Build history of the part. All positions in model axes, mm. A direction names the side the tool comes from. Give positions to 0.01 mm unless a question says otherwise; leave off trailing zeros. Loops run counter-clockwise (first coordinate to the right, second up) from the corner with the lowest first, then second, coordinate; pieces in that order, holes last.
1) Band-saw the part on C-C on y = 1. List the corners of the cut face in (x, z), then the cut area to 3 significant figures.
2) Flat gauge pin, fed straight in: P1, Ø5.5, axis at x = -3.5, y = -0.5, coming from the +Z side. Where does the tip first touch, or does it go through?
3) Band-saw the part on B-B on x = 4.5. List the corners of the cut face in (y, z).
4) Band-saw the part on D-D on z = 6.75. List the corners of the cut face in (x, y).
5) 3-axis set-ups, long thin cutter, end or side, ignore diameter. For faces 4 (the cylindrical face through (9.644, 6.124, 4.19)), 5 (the flat face through (-8.5, 0, 4)): which of +Z, -Z, +X, -X, +Y, -Y reach the whole face in a straight line?
6) Two-plate mould, pull along Y, no slides. Class faces 1 (the cylindrical face through (-9.644, -6.124, 4.19)), 2 (the flat face through (0, -5, 4)), 3 (the flat face through (0, 6.5, 4)): +Y half, -Y half, draft (parallel to the pull), parting line (faces both ways), or undercut.
7) Band-saw the part on A-A on z = 4.25. List the corners of the cut face in (x, y), then the cut area to 3 significant figures.
8) Wall check: line 1 (Y direction, x = -6, z = 8.25); line 2 (X direction, y = -2, z = 7.75); line 3 (X direction, y = 4.75, z = 3.75). Give the ranges that are in metal, low to high.
```python
from build123d import *

# Parameters (mm, degrees)
F1_DEPTH = 1.5
F3_DEPTH = 7
F5_DEPTH = 2


with BuildPart() as f1:
    # F0 (on Top) → F1 (new body)
    with BuildSketch(Plane.XY):
        with BuildLine():
            Line((8.75, 6.5), (-8.75, 6.5))
            ThreePointArc((-8.75, 6.5), (-9.633883, 6.133883), (-10, 5.25))
            Line((-10, 5.25), (-10, -5.25))
            ThreePointArc((-10, -5.25), (-9.633883, -6.133883), (-8.75, -6.5))
            Line((-8.75, -6.5), (8.75, -6.5))
            ThreePointArc((8.75, -6.5), (9.633883, -6.133883), (10, -5.25))
            Line((10, -5.25), (10, 5.25))
            ThreePointArc((10, 5.25), (9.633883, 6.133883), (8.75, 6.5))
        make_face()
    extrude(amount=F1_DEPTH)

    # F2 (on face) → F3 (join)
    with BuildSketch(Plane.XY.offset(1.5)):
        with BuildLine():
            ThreePointArc((10, 5.25), (9.633883, 6.133883), (8.75, 6.5))
            Line((8.75, 6.5), (-8.75, 6.5))
            ThreePointArc((-8.75, 6.5), (-9.633883, 6.133883), (-10, 5.25))
            Line((-10, 5.25), (-10, -5.25))
            ThreePointArc((-10, -5.25), (-9.633883, -6.133883), (-8.75, -6.5))
            Line((-8.75, -6.5), (8.75, -6.5))
            ThreePointArc((8.75, -6.5), (9.633883, -6.133883), (10, -5.25))
            Line((10, -5.25), (10, 5.25))
        make_face()
        with BuildLine():
            ThreePointArc((-8.5, 3.75), (-8.133883, 4.633883), (-7.25, 5))
            Line((-7.25, 5), (7.25, 5))
            ThreePointArc((7.25, 5), (8.133883, 4.633883), (8.5, 3.75))
            Line((8.5, 3.75), (8.5, -3.75))
            ThreePointArc((8.5, -3.75), (8.133883, -4.633883), (7.25, -5))
            Line((7.25, -5), (-7.25, -5))
            ThreePointArc((-7.25, -5), (-8.133883, -4.633883), (-8.5, -3.75))
            Line((-8.5, -3.75), (-8.5, 3.75))
        make_face(mode=Mode.SUBTRACT)
    extrude(amount=F3_DEPTH)

    # F4 (on face) → F5 (cut)
    with BuildSketch(Plane.XY.offset(8.5)):
        with BuildLine():
            Line((8, 5.5), (-8, 5.5))
            ThreePointArc((-8, 5.5), (-8.707107, 5.207107), (-9, 4.5))
            Line((-9, 4.5), (-9, -4.5))
            ThreePointArc((-9, -4.5), (-8.707107, -5.207107), (-8, -5.5))
            Line((-8, -5.5), (8, -5.5))
            ThreePointArc((8, -5.5), (8.707107, -5.207107), (9, -4.5))
            Line((9, -4.5), (9, 4.5))
            ThreePointArc((9, 4.5), (8.707107, 5.207107), (8, 5.5))
        make_face()
    extrude(amount=-F5_DEPTH, mode=Mode.SUBTRACT)


solid = f1.part
```
Findings below:
1. outline: (-10, 0) - (10, 0) - (10, 8.5) - (9, 8.5) - (9, 6.5) - (8.5, 6.5) - (8.5, 1.5) - (-8.5, 1.5) - (-8.5, 6.5) - (-9, 6.5) - (-9, 8.5) - (-10, 8.5) - close
1. area: 49.0 mm2
2. P1: stops at z = 1.5
3. outline: (-6.5, 0) - (6.5, 0) - (6.5, 8.5) - (5.5, 8.5) - (5.5, 6.5) - (5, 6.5) - (5, 1.5) - (-5, 1.5) - (-5, 6.5) - (-5.5, 6.5) - (-5.5, 8.5) - (-6.5, 8.5) - close
4. outline: (-10, -5.25) arc R1.25 ccw to (-8.75, -6.5) - (8.75, -6.5) arc R1.25 ccw to (10, -5.25) - (10, 5.25) arc R1.25 ccw to (8.75, 6.5) - (-8.75, 6.5) arc R1.25 ccw to (-10, 5.25) - close; hole (-9, -4.5) arc R1 ccw to (-8, -5.5) - (8, -5.5) arc R1 ccw to (9, -4.5) - (9, 4.5) arc R1 ccw to (8, 5.5) - (-8, 5.5) arc R1 ccw to (-9, 4.5) - close
5. face 4: +Z, -Z, +X, +Y
5. face 5: +Z
6. face 1: -Y half
6. face 2: undercut
6. face 3: +Y half
7. outline: (-10, -5.25) arc R1.25 ccw to (-8.75, -6.5) - (8.75, -6.5) arc R1.25 ccw to (10, -5.25) - (10, 5.25) arc R1.25 ccw to (8.75, 6.5) - (-8.75, 6.5) arc R1.25 ccw to (-10, 5.25) - close; hole (-8.5, -3.75) arc R1.25 ccw to (-7.25, -5) - (7.25, -5) arc R1.25 ccw to (8.5, -3.75) - (8.5, 3.75) arc R1.25 ccw to (7.25, 5) - (-7.25, 5) arc R1.25 ccw to (-8.5, 3.75) - close
7. area: 90.0 mm2
8. line 1: y = -6.5 to -5.5, 5.5 to 6.5
8. line 2: x = -10 to -9, 9 to 10
8. line 3: x = -10 to -8, 8 to 10
